from build123d import *

# Parameters (mm, degrees)
SKETCH1_W           = 4.1783
SKETCH1_H           = 8.0391
SKETCH1_W_2         = 5.588
SKETCH1_H_2         = 15.0876
SKETCH1_W_3         = 13.843
SKETCH1_H_3         = 3.048
SKETCH1_R           = 2.96545
BOSS_EXTRUDE1_DEPTH = 3.048


with BuildPart() as part:
    # Sketch1 → Boss-Extrude1 (new body)
    with BuildSketch(Plane.XY):
        Polygon((3.175, 64.77), (3.175, 53.213), (0, 53.213), (0, 6.35), (3.175, 6.35), (3.175, -3.048), (5.715, -3.048), (5.715, 0), (19.558, 0), (19.558, -3.048), (22.098, -3.048), (22.098, 3.2766), (25.273, 3.2766), (25.273, 63.754), (22.098, 63.754), (22.098, 68.834), (0, 68.834), (0, 64.77), align=None)
        with Locations((19.52625, 10.64895)):
            Rectangle(SKETCH1_W, SKETCH1_H, mode=Mode.SUBTRACT)
        with Locations((17.1069, 31.8008)):
            Rectangle(SKETCH1_W_2, SKETCH1_H_2, mode=Mode.SUBTRACT)
        with Locations((12.6365, 66.294)):
            Rectangle(SKETCH1_W_3, SKETCH1_H_3, mode=Mode.SUBTRACT)
        with Locations((17.64665, 53.48605)):
            Circle(SKETCH1_R, mode=Mode.SUBTRACT)
    extrude(amount=BOSS_EXTRUDE1_DEPTH)


solid = part.part
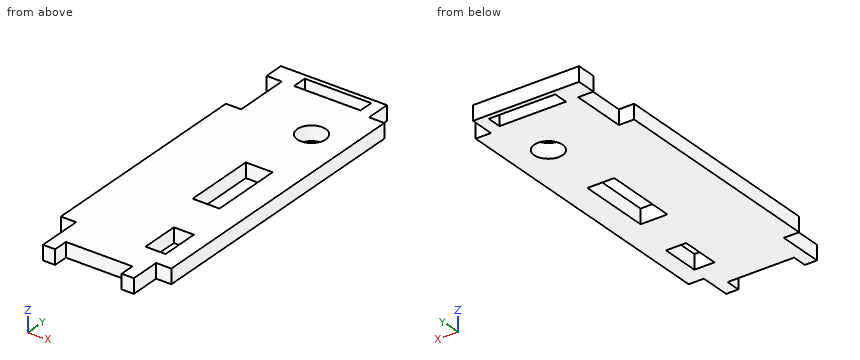
Verification items for the finished model (mm, model axes). Give positions to 0.01 mm unless a question says otherwise; leave off trailing zeros. Order: outer loops, then holes, each group sorted by start corner. A loop starts at its lowest first (then second) coordinate and runs counter-clockwise, first axis right, second up. Notation, with made-up numbers: M 54.5,34.25 L 98.5,34.25 A18 cw 98.5,56.25 Z; hole C -11.5,-24.5 d3. An arc over 180 degrees is marked long. Use one line per item in the form item = value. Start each with the question number.
Q1. Section check C-C (x = 18.75). Enter the section's corners in (y, z).
Q2. Section check D-D (z = 2.4). Count the separate pieces of the cut face and the enclosed holes in it, then the cut area to 3 significant figures.
Q3. Section check A-A (y = 7.5). Enter the section's corners in (x, z), then the cut area to 3 significant figures.
Q4. Go/stop test with flat-tipped pins: pin 1 Ø1.5 at (y, z) = (2.5, 2) entering from -X (3 decimals); pin 2 Ø1.5 at (y, z) = (67.5, 2) entering from +X; pin 3 Ø1.5 at (x, z) = (10, 2) entering from -Y. Record where each tip stops, or that it passes through.
Q5. Scan lines: line 1 along Y through (x, z) = (17.5, 1.1); line 2 along X through (y, z) = (31, 1.35); line 3 along Y through (x, z) = (8.5, 2.45). Record each from-to range of solid material in increasing order. Write a range as [from, to].
Q6. Section check B-B (x = 2.25). Enter the section's corners in (y, z).
Evaluation:
q1.outline = M 0,0 L 6.63,0 L 6.63,3.05 L 0,3.05 Z; M 14.67,0 L 24.26,0 L 24.26,3.05 L 14.67,3.05 Z; M 39.34,0 L 50.73,0 L 50.73,3.05 L 39.34,3.05 Z; M 56.24,0 L 64.77,0 L 64.77,3.05 L 56.24,3.05 Z; M 67.82,0 L 68.83,0 L 68.83,3.05 L 67.82,3.05 Z
q2.separate_pieces = 1
q2.enclosed_holes = 4
q2.area = 1,480 mm2
q3.outline = M 0,0 L 17.44,0 L 17.44,3.05 L 0,3.05 Z; M 21.62,0 L 25.27,0 L 25.27,3.05 L 21.62,3.05 Z
q3.area = 64.3 mm2
q4.pin_1 = 3.175
q4.pin_2 = 22.1
q4.pin_3 = 0
q5.line_1 = [0, 6.63], [14.67, 24.26], [39.34, 50.52], [56.45, 64.77], [67.82, 68.83]
q5.line_2 = [0, 14.31], [19.9, 25.27]
q5.line_3 = [0, 64.77], [67.82, 68.83]
q6.outline = M 6.35,0 L 53.21,0 L 53.21,3.05 L 6.35,3.05 Z; M 64.77,0 L 68.83,0 L 68.83,3.05 L 64.77,3.05 Z
